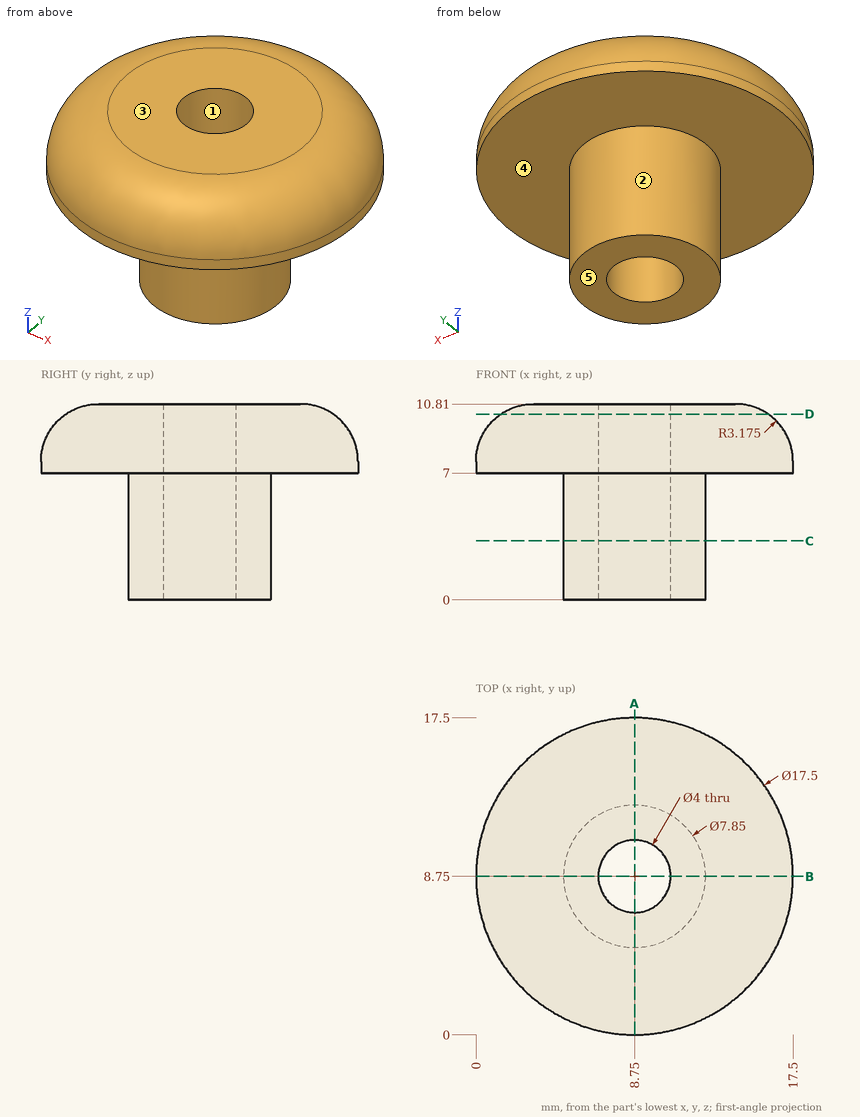
Input: dimensioned drawing with shaded views. Units: mm. Origin: part minimum x, y, z. A direction names the side the tool comes from. Give positions to 0.01 mm unless a question says otherwise; leave off trailing zeros. Order: outer loops, then holes, each group sorted by start corner. A loop starts at its lowest first (then second) coordinate and runs counter-clockwise, first axis right, second up. Notation, with made-up numbers: (40, 17.5) -> (67, 17.5) arc R22 cw to (67, 42.5) -> close; hole circle Ø9 at (12.5, -39). An arc over 180 degrees is marked (long way). Use one line per item in the form item = value.
1) Reachability of the marked faces 4 and 5 from +Z, -Z, +X, -X, +Y, -Y: full face, straight path, thin tool, end or side. Return the list, or none.
Response values:
face_4 = -Z
face_5 = -Z, +X, -X, +Y, -Y
2) First-contact query: pin 1 Ø1.5 at (x, z) = (6.5, 9.5) entering from -Y; pin 2 Ø3 at (y, z) = (11.5, 7) entering from +X; pin 3 Ø4 at (x, z) = (9.5, 1.5) entering from +Y (3 decimals). Flat tips, straight axial feed; report the tip coordinate or a pass-through.
Response values:
pin_1 = 0.45
pin_2 = 17.41
pin_3 = 12.675
3) Section C-C, the plane z = 3.25. Return loops of the section in (x, y) (3 decimals).
Response values:
outline = circle Ø7.85 at (8.75, 8.75); hole circle Ø4 at (8.75, 8.75)
4) Section A-A, the plane x = 8.75. Return loops of the section in (y, z) (3 decimals), and give its area (3 significant figures).
Response values:
outline = (0, 7) -> (4.825, 7) -> (4.825, 0) -> (6.75, 0) -> (6.75, 10.81) -> (3.175, 10.81) arc R3.175 ccw to (0, 7.635) -> close; (10.75, 0) -> (12.675, 0) -> (12.675, 7) -> (17.5, 7) -> (17.5, 7.635) arc R3.175 ccw to (14.325, 10.81) -> (10.75, 10.81) -> close
area = 74.1 mm^2
5) Section D-D, the plane z = 10.25. Return loops of the section in (x, y), and give its area (3 significant figures).
Response values:
outline = circle Ø14.75 at (8.75, 8.75); hole circle Ø4 at (8.75, 8.75)
area = 158 mm^2
6) Mould query, pull axis X, two halves, no side actions, for the marked faces 1, 2 and 3. Classes: pulls with the +X half, pulls with the -X half, needs draft (parallel to the pull), parting line crosses it, or undercut.
Response values:
face_1 = undercut
face_2 = parting line crosses it
face_3 = needs draft
7) Line query: probe 1 along Y at (x, z) = (8.75, 7.75); probe 2 along Y at (x, z) = (8.75, 3.5) (3 decimals); probe 3 along Z at (x, y) = (14.5, 9). Output: solid intervals per line, ascending.
Response values:
probe_1 = 0 to 6.75, 10.75 to 17.5
probe_2 = 4.825 to 6.75, 10.75 to 12.675
probe_3 = 7 to 10.8
